Autodesk Fusion 360 part; units mm, degrees
sketch "Sketch1" plane through (0, 0, 0) normal (0, 0, 1) x (1, 0, 0)
  line L0 (0.5, 3.925) -> (8.0469, 3.925)
  line L1 (7.9531, 3.575) -> (0.5, 3.575)
  line L2 (0.5, 3.575) -> (0.5, 3.925)
  line L3 (0.5, 3.75) -> (8, 3.75) construction
  line L4 (8, 3.75) -> (14.4952, 0) construction
  line L5 (8.0469, 3.925) -> (14.5827, 0.1516)
  line L6 (14.5827, 0.1516) -> (14.4077, -0.1516)
  line L7 (14.4077, -0.1516) -> (7.9531, 3.575)
  dimension "d1" = 150
  dimension "d2" = 0.35
  dimension "d3" = 0.35
  dimension "d14" = 7.5
  dimension "d15" = 7.5
  dimension "d16" = 3.75
  dimension "d20" = 0.5
extrude "Extrude1" add sketch "Sketch1" along normal blind 0.35
equation "d1 = angle"
equation "d2 = channelwidth"
equation "d3 = d2"
equation "angle = 150 deg"
equation "channelwidth = 0.35 mm"
equation "length = 7.5 mm"
equation "length2 = 7.5 mm"
equation "depth = 0.35 mm"
equation "d11 = depth"
equation "d14 = length2"
equation "d15 = length"
equation "d16 = yoffset"
equation "yoffset = length2 * cos(angle - 90 deg)"
equation "xoffset = 0.5 mm"
equation "d20 = xoffset"
Work out the finished part from the listing and answer in its coordinate system (mm). Round coordinates to 2 decimals unless told otherwise and drop trailing zeros. Loops run counter-clockwise (first coordinate to the right, second up) from the corner with the lowest first, then second, coordinate; pieces in that order, holes last. Notation, with made-up numbers: (53.5, 24) -> (99.5, 24) arc R21 ccw to (99.5, 57) -> close; hole circle Ø10 at (8.25, 39). An arc over 180 degrees is marked (long way). Write each question's results on one line, items separated by ' | '. Start each with the question number.
1. Find the intervals of material crossed by probe 1 along Y at (x, z) = (3.5, 0.05) (3 decimals); probe 2 along Y at (x, z) = (9.25, 0.1); probe 3 along X at (y, z) = (2.2, 0.1), in increasing order. Write a range as from..to.
2. Section A-A (z = 0.2) is taken. Determine the outline of the cut face in (x, y) (3 decimals), plus the area to 3 significant figures.
3. Section B-B (x = 3) is taken. Determine the outline of the cut face in (y, z) (3 decimals), plus the area to 4 significant figures.
4. Section C-C (y = 2.85) is taken. Determine the outline of the cut face in (x, z), plus the area to 3 significant figures.
Evaluation:
1) probe 1: y = 3.575..3.925 | probe 2: y = 2.83..3.23 | probe 3: x = 10.33..11.03
2) outline: (0.5, 3.575) -> (7.953, 3.575) -> (14.408, -0.152) -> (14.583, 0.152) -> (8.047, 3.925) -> (0.5, 3.925) -> close | area: 5.25 mm2
3) outline: (3.575, 0) -> (3.925, 0) -> (3.925, 0.35) -> (3.575, 0.35) -> close | area: 0.1225 mm2
4) outline: (9.21, 0) -> (9.91, 0) -> (9.91, 0.35) -> (9.21, 0.35) -> close | area: 0.245 mm2
